Read the model definition and answer for the solid it produces. Units are mm, in the model's axes. A direction names the side the tool comes from. Coordinates: 2 decimals unless noted, no trailing zeros. Order: outer loops, then holes, each group sorted by start corner. A loop starts at its lowest first (then second) coordinate and runs counter-clockwise, first axis right, second up. Notation, with made-up numbers: (9, 32.25) -> (53, 32.25) arc R19 ccw to (53, 64.25) -> close; hole circle Ø5 at (85, -15). An arc over 180 degrees is marked (long way). Answer in a Markdown table with one row per item.
from build123d import *

# Parameters (mm, degrees)
SKETCH1_R           = 40
BOSS_EXTRUDE1_DEPTH = 100
SKETCH3_W           = 54.17424305
SKETCH3_H           = 80
CUT_EXTRUDE1_DEPTH  = 158.797338381
HOLE1_D             = 20
FILLET1_R           = 10
SKETCH6_W           = 45
SKETCH6_H           = 15
SKETCH6_H_2         = 30


with BuildPart() as part:
    # Sketch1 → Boss-Extrude1 (new body)
    with BuildSketch(Plane(origin=(0, 0, 0), x_dir=(1, 0, 0), z_dir=(0, 1, 0))):
        with BuildLine():
            Line((45.82575695, 20), (100, 20))
            Line((100, 20), (100, -20))
            Line((100, -20), (45.82575695, -20))
            ThreePointArc((45.82575695, -20), (0, -50), (-45.82575695, -20))
            Line((-45.82575695, -20), (-100, -20))
            Line((-100, -20), (-100, 20))
            Line((-100, 20), (-45.82575695, 20))
            ThreePointArc((-45.82575695, 20), (0, 50), (45.82575695, 20))
        make_face()
        with Locations(Location((0, 0, 0), (0, 0, 270))):
            Circle(SKETCH1_R, mode=Mode.SUBTRACT)
    extrude(amount=BOSS_EXTRUDE1_DEPTH)

    # Sketch3 → Cut-Extrude1 (cut, symmetric)
    with BuildSketch(Plane.XY.offset(20)):
        with Locations((72.912878475, 50)):
            Rectangle(SKETCH3_W, SKETCH3_H)
    cut_extrude1 = extrude(amount=CUT_EXTRUDE1_DEPTH, both=True, mode=Mode.SUBTRACT)

    # Mirror1: Cut-Extrude1 across plane
    add(cut_extrude1.mirror(Plane(origin=(0, 0, 0), x_dir=(0, 0, 1), z_dir=(1, 0, 0))), mode=Mode.SUBTRACT)

    # Hole1 (through all)
    with Locations(Plane(origin=(0, 100, 0), x_dir=(1, 0, 0), z_dir=(0, 1, 0))):
        with Locations((-75, 0), (75, 0)):
            Hole(HOLE1_D / 2)

    # Fillet1
    fillet1_edges = [part.edges().sort_by_distance(p)[0] for p in [
        (100, 95, 20),
        (-100, 95, 20),
        (-100, 95, -20),
        (100, 95, -20),
        (100, 5, 20),
        (100, 5, -20),
        (-100, 5, 20),
        (-100, 5, -20),
    ]]
    fillet(fillet1_edges, radius=FILLET1_R)

    # Sketch6 → Cut-Revolve1 (revolve, cut)
    with BuildSketch(Plane.XY, mode=Mode.PRIVATE) as cut_revolve1_sk:
        with Locations((22.5, 82.5)):
            Rectangle(SKETCH6_W, SKETCH6_H)
        with Locations((22.5, 50)):
            Rectangle(SKETCH6_W, SKETCH6_H_2)
        with Locations((22.5, 17.5)):
            Rectangle(SKETCH6_W, SKETCH6_H)
    revolve(cut_revolve1_sk.sketch.rotate(Axis((0, 0, 0), (0, 1, 0)), 90), axis=Axis((0, 0, 0), (0, 1, 0)), mode=Mode.SUBTRACT)


solid = part.part
Q1. For faces 1 (the face through (68, 95, -20)), 2 (the face through (68, 5, 20)), 3 (the face through (26.5, 25, -30.2)), 4 (the face through (-67, 10, -9)), determine the directions among +Z, -Z, +X, -X, +Y, -Y from which every point of the face is accessible in a straight line to the end or side of a thin tool.
Outcome:
| item | result |
|---|---|
| face 1 | -Z, +X, +Y, -Y |
| face 2 | +Z, +X, +Y, -Y |
| face 3 | none |
| face 4 | +Z, -Z, -X |
Q2. The part is cut by section B-B (y = 42). Write down the section's boundary in (x, z).
Outcome:
| item | result |
|---|---|
| outline | (-45.83, -20) arc R50 ccw to (45.83, -20) -> (45.83, 20) arc R50 ccw to (-45.83, 20) -> close; hole circle Ø90 at (0, 0) |
Q3. Given pin 1 (1.5 mm diameter, centred on y = 30.5, z = 29.5, fed in from -X); pin 2 (8 mm diameter, centred on x = 60.5, y = 7.5, fed in from -Z); pin 3 (6 mm diameter, centred on x = 46, y = 12, fed in from +Z), each flat-ended and moving along its own axis, determine where each tip first touches the part or whether it passes through.
Outcome:
| item | result |
|---|---|
| pin 1 | x = -40.91 |
| pin 2 | z = -20 |
| pin 3 | z = 25.51 |
Q4. Consider line 1 (Y direction, x = -22.5, z = 35); line 2 (X direction, y = 14, z = 0); line 3 (X direction, y = 29.5, z = 0). Determine where each line is inside the solid, lowest interval first.
Outcome:
| item | result |
|---|---|
| line 1 | 0 to 10, 25 to 35, 65 to 75, 90 to 100 |
| line 2 | -45.83 to -45, 45 to 45.83 |
| line 3 | -45.83 to -40, 40 to 45.83 |
Q5. For a pull along X with two mould halves and no side action, classify faces 5 (the face through (-39.05, 69.93, -8.67)), 6 (the face through (-45.826, 49, 0)), 7 (the face through (-67, 90, -9)) as pulls with the +X half, pulls with the -X half, needs draft (parallel to the pull), parting line crosses it, or undercut.
Outcome:
| item | result |
|---|---|
| face 5 | undercut |
| face 6 | pulls with the -X half |
| face 7 | needs draft |
Q6. The part is cut by section D-D (x = 75). Write down the section's boundary in (y, z), then the cut area to 3 significant figures.
Outcome:
| item | result |
|---|---|
| outline | (0, -20) -> (10, -20) -> (10, -10) -> (0, -10) -> close; (0, 10) -> (10, 10) -> (10, 20) -> (0, 20) -> close; (90, -20) -> (100, -20) -> (100, -10) -> (90, -10) -> close; (90, 10) -> (100, 10) -> (100, 20) -> (90, 20) -> close |
| area | 400 mm² |
Q7. The part is cut by section A-A (x = -55). Write down the section's boundary in (y, z).
Outcome:
| item | result |
|---|---|
| outline | (0, -20) -> (10, -20) -> (10, 20) -> (0, 20) -> close; (90, -20) -> (100, -20) -> (100, 20) -> (90, 20) -> close |
